Work out the finished part from the listing and answer in its coordinate system (mm). Coordinates: 2 decimals unless noted, no trailing zeros. Order: outer loops, then holes, each group sorted by start corner. A loop starts at its lowest first (then second) coordinate and runs counter-clockwise, first axis right, second up.
1. The part is cut by section B-B, the plane y = 12.7. Give the vertices of the cut face in (x, z).
2. The part is cut by section C-C, the plane z = 1.1. Count the separate pieces of the cut face and the enclosed holes in it, then the cut area to 3 significant figures.
3. Find the intervals of material crossed by probe 1 along Y at (x, z) = (6.35, 0.6); probe 2 along X at (y, z) = (78, 0.65); probe 3 along X at (y, z) = (71, 1.05), in increasing order.
4. The part is cut by section D-D, the plane x = 30.5. Give the vertices of the cut face in (y, z), then the cut area to 3 significant figures.
5. The part is cut by section A-A, the plane x = 19.05. Give the vertices of the cut face in (y, z).
Autodesk Inventor part; units mm, degrees
ref_plane "YZ Plane" through (0, 0, 0) normal (1, 0, 0) x (0, 1, 0)
ref_plane "XZ Plane" through (0, 0, 0) normal (0, 1, 0) x (-1, 0, 0)
ref_plane "XY Plane" through (0, 0, 0) normal (0, 0, 1) x (1, 0, 0)
sketch "Sketch1" plane through (0, 0, 0) normal (0, 0, 1) x (1, 0, 0)
  line L0 (106.3625, -44.45) -> (0, -44.45)
  line L1 (110.551814, -19.05) -> (110.551814, -44.45)
  line L2 (106.3625, -19.05) -> (110.551814, -19.05)
  line L3 (106.3625, -19.05) -> (110.551814, -19.05)
  line L4 (110.551814, -19.05) -> (110.551814, -22.225)
  line L5 (110.551814, -22.225) -> (106.3625, -22.225)
  line L6 (106.3625, -22.225) -> (106.3625, -19.05)
  line L7 (106.3625, -19.05) -> (106.3625, -44.45)
  line L8 (110.551814, -19.05) -> (110.551814, -44.45)
  line L9 (106.3625, -41.275) -> (110.551814, -41.275)
  line L10 (110.551814, -41.275) -> (110.551814, -44.45)
  line L11 (110.551814, -44.45) -> (106.3625, -44.45)
  line L12 (106.3625, -44.45) -> (106.3625, -41.275)
  point P0 (0, 0)
  point P1 (110.551814, -34.925)
  point P2 (111.304505, 0)
  point P3 (131.506814, -44.45)
  point P4 (131.506814, -19.05)
  dimension "d6" = 25.4
  dimension "d22" = 12.7
  dimension "d54" = 25.4
  dimension "d55" = 106.3625
  dimension "d56" = 25.4
  dimension "d57" = 44.45
  dimension "d58" = 9.525
  dimension "d81" = 6.35
  dimension "d82" = 6.35
  dimension "d85" = 12.7
  dimension "d88" = 12.7
sketch "Sketch1 outline for Plate1" plane through (0, 0, 0) normal (0, 0, 1) x (1, 0, 0)
  line L0 (0, 106.3625) -> (0, 0)
  line L1 (25.4, 106.3625) -> (0, 106.3625)
  line L2 (0, 0) -> (44.45, 0)
  line L3 (44.45, 25.4) -> (25.4, 106.3625)
  line L4 (44.45, 0) -> (44.45, 25.4)
  circle A0 centre (9.525, 12.7) radius 2.0701
  circle A1 centre (34.925, 12.7) radius 2.0701
  circle A2 centre (6.35, 87.3125) radius 2.0701
  circle A3 centre (6.35, 100.0125) radius 2.0701
  circle A4 centre (19.05, 87.3125) radius 2.0701
  circle A5 centre (19.05, 100.0125) radius 2.0701
extrude "Plate1" add sketch "Sketch1 outline for Plate1" along normal blind 1.5875
ref_plane "Work Plane1" through (0, 110.8075, 25.4) normal (0, 1, 0) x (1, 0, 0)
sketch "Sketch4 outline for Cut3" plane through (0, 110.8075, 25.4) normal (0, 1, 0) x (1, 0, 0)
  line L0 (0, 20.955) -> (0, 0)
  line L1 (0, 0) -> (25.4, 0)
  line L2 (25.4, 0) -> (25.4, 20.955)
  line L3 (25.4, 20.955) -> (0, 20.955)
extrude "Cut3" cut sketch "Sketch4 outline for Cut3" against normal blind 1.5875
fillet "Fillet5" radius 12.7 1 edges at (44.45, 25.4, 0.7937)
sketch "Sketch4" plane through (0, 110.8075, 25.4) normal (0, 1, 0) x (1, 0, 0)
  line L0 (25.4, 0) -> (0, 0)
  circle A0 centre (19.05, 6.35) radius 2.3749
  line L1 (0, 0) -> (0, 20.955)
  line L2 (0, 20.955) -> (25.4, 20.955)
  line L3 (25.4, 20.955) -> (25.4, 21.413463)
  line L4 (21.135301, 0) -> (22.225, 0)
  line L5 (0, 0) -> (0, 20.955)
  line L6 (25.4, 20.955) -> (0, 20.955)
  line L7 (25.4, 20.955) -> (25.4, 17.78)
  line L8 (25.4, 17.78) -> (25.4, 9.525)
  line L9 (12.7, 9.525) -> (12.7, 20.955)
  arc A1 (12.7, 9.525) -> (22.225, 0) centre (22.225, 9.525) ccw
  line L10 (25.4, 20.955) -> (25.4, 0)
  line L11 (0, 0) -> (25.4, 0)
  line L12 (25.4, 0) -> (25.4, 20.955)
  point P0 (0, 25.4)
  point P1 (12.7, 0)
  point P2 (25.4, 0)
  point P3 (12.7, 0)
  dimension "d28" = 4.7498
  dimension "d29" = 6.35
  dimension "d34" = 19.05
  dimension "d47" = 3.175
  dimension "d48" = 6.35
  dimension "d49" = 6.35
  dimension "d50" = 9.525
equation "\"d51\" = Thickness"
equation "\"BendRadius\" = Thickness"
equation "\"BendReliefWidth\" = Thickness"
equation "\"BendReliefDepth\" = 0.5 * Thickness"
equation "\"CornerReliefSize\" = 4 * Thickness"
equation "\"MinimumRemnant\" = 2 * Thickness"
equation "\"TransitionRadius\" = BendRadius"
equation "\"JacobiRadiusSize\" = BendRadius"
equation "\"GapSize\" = Thickness"
equation "\"d11\" = BendRadius"
properties part number "Pneumatic Piston Front Flange (Left Custom)" material "Aluminum 6061"
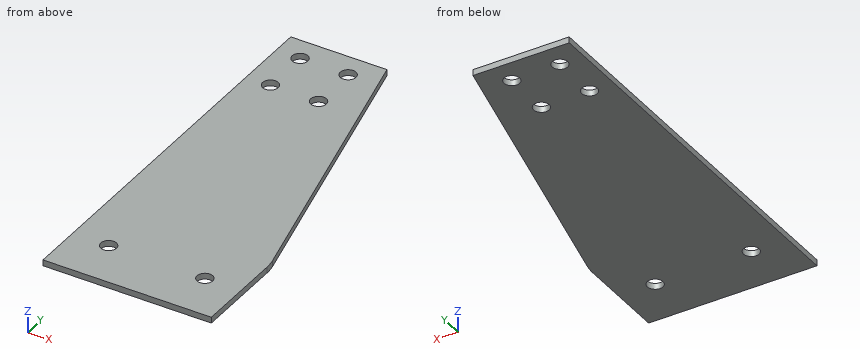
Geometry says:
1. outline: (0, 0) - (7.45, 0) - (7.45, 1.59) - (0, 1.59) - close; (11.6, 0) - (32.85, 0) - (32.85, 1.59) - (11.6, 1.59) - close; (37, 0) - (44.45, 0) - (44.45, 1.59) - (37, 1.59) - close
2. separate pieces: 1
2. enclosed holes: 6
2. area: 3,880 mm2
3. probe 1: y = 0 to 85.24, 89.38 to 97.94, 102.08 to 106.36
3. probe 2: x = 0 to 32.07
3. probe 3: x = 0 to 33.72
4. outline: (0, 0) - (84.69, 0) - (84.69, 1.59) - (0, 1.59) - close
4. area: 134 mm2
5. outline: (0, 0) - (85.24, 0) - (85.24, 1.59) - (0, 1.59) - close; (89.38, 0) - (97.94, 0) - (97.94, 1.59) - (89.38, 1.59) - close; (102.08, 0) - (106.36, 0) - (106.36, 1.59) - (102.08, 1.59) - close
